```python
from build123d import *

# Parameters (mm, degrees)
EXTRUDE_1_DEPTH     = 4.5
EXTRUDE_2_DEPTH     = 7.4
SKETCH_3_R          = 11
EXTRUDE_3_DEPTH     = 4
CUT_EXTRUDE_2_REACH = 77.071
SKETCH_7_R          = 1.75
SKETCH_10_R         = 1.478021834
SKETCH_10_W         = 41
SKETCH_10_H         = 21
CUT_EXTRUDE_3_DEPTH = 14
SKETCH_12_R         = 5.390059672
CUT_EXTRUDE_4_DEPTH = 15


with BuildPart() as part:
    # 草图1 → 凸台-拉伸1 (new body)
    with BuildSketch(Plane.XY):
        with BuildLine():
            Line((-52.25, 0), (52.25, 0))
            ThreePointArc((52.25, 0), (0, -52.25), (-52.25, 0))
        make_face()
    extrude(amount=EXTRUDE_1_DEPTH)

    # 草图2 → 凸台-拉伸2 (add, symmetric)
    with BuildSketch(Plane.XY.offset(2.25)):
        with BuildLine():
            Line((-52.25, 0), (52.25, 0))
            ThreePointArc((52.25, 0), (52.22844668, -1.500619011), (52.163804501, -3))
            Line((52.163804501, -3), (-52.163804501, -3))
            ThreePointArc((-52.163804501, -3), (-52.22844668, -1.500619011), (-52.25, 0))
        make_face()
    extrude(amount=EXTRUDE_2_DEPTH, both=True)

    # 草图3 → 凸台-拉伸3 (add)
    with BuildSketch(Plane(origin=(0, -52.25, 0), x_dir=(1, 0, 0), z_dir=(0, 1, 0))):
        with Locations(Location((0, -2.25, 0), (0, 0, 168.19710831))):
            Circle(SKETCH_3_R)
    extrude(amount=EXTRUDE_3_DEPTH)

    # 草图7 → 切除-拉伸2 (cut, up to next)
    with BuildSketch(Plane.XZ.offset(52.25), mode=Mode.PRIVATE) as cut_extrude_2_sk1:
        with Locations(Location((0, 9.25, 0), (0, 0, 270))):
            Circle(SKETCH_7_R)
    cut_extrude_2_tool1 = extrude(cut_extrude_2_sk1.sketch, amount=-CUT_EXTRUDE_2_REACH, mode=Mode.PRIVATE) & part.part
    # 草图7 → 切除-拉伸2 (cut, up to next)
    with BuildSketch(Plane.XZ.offset(52.25), mode=Mode.PRIVATE) as cut_extrude_2_sk2:
        with Locations(Location((0, -4.75, 0), (0, 0, 270))):
            Circle(SKETCH_7_R)
    cut_extrude_2_tool2 = extrude(cut_extrude_2_sk2.sketch, amount=-CUT_EXTRUDE_2_REACH, mode=Mode.PRIVATE) & part.part
    add(cut_extrude_2_tool1.solids().sort_by_distance((0, -52.25, 9.25))[0], mode=Mode.SUBTRACT)
    add(cut_extrude_2_tool2.solids().sort_by_distance((0, -52.25, -4.75))[0], mode=Mode.SUBTRACT)

    # 草图10 → 切除-拉伸3 (cut)
    with BuildSketch(Plane.XY.offset(4.5)):
        with Locations((-14.143943937, -23.76680221)):
            Circle(SKETCH_10_R)
        with Locations((34.286056063, -23.76680221)):
            Circle(SKETCH_10_R)
        with Locations((-14.143943937, -33.76680221)):
            Circle(SKETCH_10_R)
        with Locations((34.356056063, -33.76680221)):
            Circle(SKETCH_10_R)
        with Locations((10.206056063, -28.76680221)):
            Rectangle(SKETCH_10_W, SKETCH_10_H)
    extrude(amount=-CUT_EXTRUDE_3_DEPTH, mode=Mode.SUBTRACT)

    # 草图12 → 切除-拉伸4 (cut)
    with BuildSketch(Plane.XY.offset(4.5)):
        with Locations((-29.445394051, -28.42542141)):
            Circle(SKETCH_12_R)
    extrude(amount=-CUT_EXTRUDE_4_DEPTH, mode=Mode.SUBTRACT)


solid = part.part
```
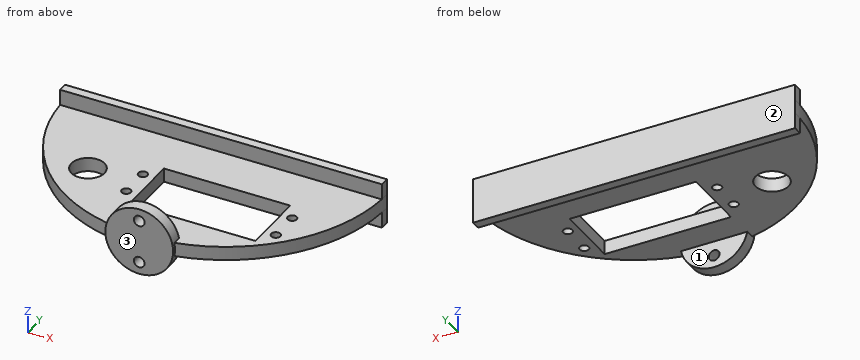
Check sheet for the modelled part. Datum: model origin and axes. Units: mm. Face numbers are marked on the shaded views. Coordinates: 2 decimals unless noted, no trailing zeros. Loops run counter-clockwise (first coordinate to the right, second up) from the corner with the lowest first, then second, coordinate; pieces in that order, holes last.
1) Sectioned sample at B-B (z = 1.75). Record the boundary of the cut face in (x, y), and give its area (3 significant figures).
2) Sectioned sample at A-A (x = 0). Record the boundary of the cut face in (y, z).
3) Release check for a two-part mould opening along Y. For the marked faces 1, 2 and 3 record: released by +Y, released by -Y, zero draft, split by the parting line, or undercut.
4) Gauge pin test, flat ends, axial feed: pin 1 (12 mm diameter, centred on y = -41.5, z = -5, fed in from -X); pin 2 (24 mm diameter, centred on x = -2.5, y = -16.5, fed in from -Z); pin 3 (2 mm diameter, centred on x = 0, z = 9.25, fed in from -Y). Record the tip position at first contact, or that the pin passes through.
5) Sectioned sample at D-D (y = -12.5). Record the boundary of the cut face in (x, z), and give its area (3 significant figures).
6) Material ranges on probe 1 along Y at (x, z) = (27, 5.5); probe 2 along X at (y, z) = (-24, 2); probe 3 along Z at (x, y) = (41, -30), recorded low to high.
7) Sectioned sample at C-C (x = -32.5). Record the boundary of the cut face in (y, z), and give its area (3 significant figures).
Check sheet entries:
1. outline: (-52.25, 0) arc R52.25 ccw to (-10.99, -51.08) - (-10.99, -52.25) - (10.99, -52.25) - (10.99, -51.08) arc R52.25 ccw to (52.25, 0) - close; hole circle Ø10.78 at (-29.45, -28.43); hole circle Ø2.96 at (-14.14, -33.77); hole circle Ø2.96 at (-14.14, -23.77); hole (-10.29, -39.27) - (30.71, -39.27) - (30.71, -18.27) - (-10.29, -18.27) - close; hole circle Ø2.96 at (34.29, -23.77); hole circle Ø2.96 at (34.36, -33.77)
1. area: 3,320 mm2
2. outline: (-52.25, -8.75) - (-48.25, -8.75) - (-48.25, -6.5) - (-52.25, -6.5) - close; (-52.25, -3) - (-48.25, -3) - (-48.25, 0) - (-39.27, 0) - (-39.27, 4.5) - (-48.25, 4.5) - (-48.25, 7.5) - (-52.25, 7.5) - close; (-52.25, 11) - (-48.25, 11) - (-48.25, 13.25) - (-52.25, 13.25) - close; (-18.27, 0) - (-3, 0) - (-3, -5.15) - (0, -5.15) - (0, 9.65) - (-3, 9.65) - (-3, 4.5) - (-18.27, 4.5) - close
3. face 1: undercut
3. face 2: released by +Y
3. face 3: released by -Y
4. pin 1: stops at x = -35.67
4. pin 2: stops at z = 0
4. pin 3: stops at y = -3
5. outline: (-50.73, 0) - (50.73, 0) - (50.73, 4.5) - (-50.73, 4.5) - close
5. area: 457 mm2
6. probe 1: y = -3 to 0
6. probe 2: x = -46.41 to -32.52, -26.37 to -15.6, -12.68 to -10.29, 30.71 to 32.83, 35.75 to 46.41
6. probe 3: z = 0 to 4.5
7. outline: (-40.91, 0) - (-32.87, 0) - (-32.87, 4.5) - (-40.91, 4.5) - close; (-23.98, 0) - (-3, 0) - (-3, -5.15) - (0, -5.15) - (0, 9.65) - (-3, 9.65) - (-3, 4.5) - (-23.98, 4.5) - close
7. area: 175 mm2
